```python
from build123d import *

# Parameters (mm, degrees)
SKETCH1_R           = 4.5
BOSS_EXTRUDE1_DEPTH = 4.5
BOSS_EXTRUDE2_START = -23
SKETCH1_3_R         = 4.5
BOSS_EXTRUDE2_DEPTH = 23
SKETCH2_R           = 9.498901539
BOSS_EXTRUDE3_DEPTH = 10
BOSS_EXTRUDE4_DEPTH = 3


with BuildPart() as part:
    # Sketch1 → Boss-Extrude1 (new body)
    with BuildSketch(Plane.XY):
        with BuildLine():
            Line((2.589777271, 3.680088815), (6.019261146, 7.349727563))
            ThreePointArc((6.019261146, 7.349727563), (0, 9.5), (-6.019261146, 7.349727563))
            Line((-6.019261146, 7.349727563), (-2.589777271, 3.680088815))
            ThreePointArc((-2.589777271, 3.680088815), (0, 4.5), (2.589777271, 3.680088815))
        make_face()
        Circle(SKETCH1_R)
        with BuildLine():
            Line((6.019261146, -7.349727563), (2.589777271, -3.680088815))
            ThreePointArc((2.589777271, -3.680088815), (0, -4.5), (-2.589777271, -3.680088815))
            Line((-2.589777271, -3.680088815), (-6.019261146, -7.349727563))
            ThreePointArc((-6.019261146, -7.349727563), (0, -9.5), (6.019261146, -7.349727563))
        make_face()
    extrude(amount=BOSS_EXTRUDE1_DEPTH)

    # Sketch1_3 → Boss-Extrude2 (add)
    with BuildSketch(Plane.XY.offset(BOSS_EXTRUDE2_START)):
        with Locations(Location((0, 0, 0), (0, 0, 125.135079602))):
            Circle(SKETCH1_3_R)
    extrude(amount=BOSS_EXTRUDE2_DEPTH)

    # Sketch2 → Boss-Extrude3 (add)
    with BuildSketch(Plane(origin=(0, 0, -23), x_dir=(-1, 0, 0), z_dir=(0, 0, -1))):
        Circle(SKETCH2_R)
    extrude(amount=-BOSS_EXTRUDE3_DEPTH)

    # Sketch2_3 → Boss-Extrude4 (add)
    with BuildSketch(Plane(origin=(0, 0, -23), x_dir=(-1, 0, 0), z_dir=(0, 0, -1))):
        with BuildLine():
            Line((-3.25, 13.360389216), (-3.25, 8.92561653))
            ThreePointArc((-3.25, 8.92561653), (0, 9.498901539), (3.25, 8.92561653))
            Line((3.25, 8.92561653), (3.25, 13.360389216))
            ThreePointArc((3.25, 13.360389216), (0, 13.75), (-3.25, 13.360389216))
        make_face()
        with BuildLine():
            ThreePointArc((3.25, -8.92561653), (0, -9.498901539), (-3.25, -8.92561653))
            Line((-3.25, -8.92561653), (-3.25, -13.360389216))
            ThreePointArc((-3.25, -13.360389216), (0, -13.75), (3.25, -13.360389216))
            Line((3.25, -13.360389216), (3.25, -8.92561653))
        make_face()
    extrude(amount=-BOSS_EXTRUDE4_DEPTH)


solid = part.part
```
Geometry: final body of the model. Coordinates: model frame, mm. A direction names the side the tool comes from. Round coordinates to 2 decimals unless told otherwise and drop trailing zeros. Order: outer loops, then holes, each group sorted by start corner. A loop starts at its lowest first (then second) coordinate and runs counter-clockwise, first axis right, second up. Notation, with made-up numbers: (9.25, 82) - (52.25, 82) arc R6 ccw to (52.25, 89) - close; hole circle Ø5 at (38.5, -24.5). An arc over 180 degrees is marked (long way). Use CSV: the item, a comma, the result in double quotes. Start each with the question number.
Q1. Material intervals for line 1 along Z through (x, y) = (0.5, 9); line 2 along Z through (x, y) = (3.5, 4.5); line 3 along Z through (x, y) = (1, -10.25), sorted ascending. Write a range as from..to.
Q2. Section query A-A (x = 0). Return loops of the section in (y, z).
Q3. First-contact query: pin 1 (1.5 mm diameter, centred on y = -11, z = 0, fed in from -X); pin 2 (1 mm diameter, centred on x = -2, z = -10.5, fed in from -Y); pin 3 (2.5 mm diameter, centred on y = -11.5, z = -21, fed in from +X); pin 4 (4 mm diameter, centred on y = 3.5, z = -7.5, fed in from +X). Flat tips, straight axial feed; report the tip coordinate or a pass-through.
Q4. Section query B-B (y = 6.5). Return loops of the section in (x, z).
Q5. Section query D-D (y = 0). Return loops of the section in (x, z).
Q6. Mould query, pull axis Y, two halves, no side actions, for faces 1 (the face through (-3.25, 11, -22)), 2 (the face through (-4.33, 5.54, 2.22)), 3 (the face through (-0.1, -9.5, 2.2)). Classes: +Y half, -Y half, draft (parallel to the pull), parting line (faces both ways), or undercut.
Q7. Access query for faces 4 (the face through (-9.06, 2.85, -18.07)), 5 (the face through (-3.25, -11, -22)), 6 (the face through (-4.1, 2.2, -13)), 7 (the face through (0.1, 9.5, 2.2)), 8 (the face through (3.25, -11, -22)). Directions: +Z, -Z, +X, -X, +Y, -Y. A direction counts if a zero-diameter tool reaches every point of the face in a straight line with its end or side. Return the directions, or none.
Q8. Section query C-C (z = 2.25). Return loops of the section in (x, y), and give its area (3 significant figures).
Result set:
1,line 1,"z = -23..-13, 0..4.5"
1,line 2,"z = -23..-13"
1,line 3,"z = -23..-20"
2,outline,"(-13.75, -23) - (13.75, -23) - (13.75, -20) - (9.5, -20) - (9.5, -13) - (4.5, -13) - (4.5, 0) - (9.5, 0) - (9.5, 4.5) - (-9.5, 4.5) - (-9.5, 0) - (-4.5, 0) - (-4.5, -13) - (-9.5, -13) - (-9.5, -20) - (-13.75, -20) - close"
3,pin 1,"passes through"
3,pin 2,"stops at y = -4.24"
3,pin 3,"stops at x = 3.25"
3,pin 4,"stops at x = 4.24"
4,outline,"(-6.93, -23) - (6.93, -23) - (6.93, -13) - (-6.93, -13) - close; (-5.23, 0) - (5.23, 0) - (5.23, 4.5) - (-5.23, 4.5) - close"
5,outline,"(-9.5, -23) - (9.5, -23) - (9.5, -13) - (4.5, -13) - (4.5, 4.5) - (-4.5, 4.5) - (-4.5, -13) - (-9.5, -13) - close"
6,face 1,"draft"
6,face 2,"undercut"
6,face 3,"-Y half"
7,face 4,"+Z"
7,face 5,"+Z, -Z, -X, -Y"
7,face 6,"none"
7,face 7,"+Z, +Y"
7,face 8,"+Z, -Z, +X, -Y"
8,outline,"(-6.02, -7.35) arc R9.5 ccw to (6.02, -7.35) - (2.59, -3.68) arc R4.5 ccw to (2.59, 3.68) - (6.02, 7.35) arc R9.5 ccw to (-6.02, 7.35) - (-2.59, 3.68) arc R4.5 ccw to (-2.59, -3.68) - close"
8,area,"156 mm2"
